```python
from build123d import *

# Parameters (mm, degrees)
F0_W     = 76.2
F0_H     = 76.2
F1_DEPTH = 127
F2_SIZE  = 5.08
F3_R     = 25.4
F4_DEPTH = 25.4
F5_R     = 5.08
F6_DEPTH = 76.2


with BuildPart() as f1:
    # F0 (on Front) → F1 (new body)
    with BuildSketch(Plane.XZ):
        Polygon((12.112662, -9.798872), (-64.087338, -9.798872), (-64.087338, -60.598872), (113.712662, -60.598872), (113.712662, -9.798872), align=None)
        with Locations((-25.987338, 28.301128)):
            Rectangle(F0_W, F0_H)
    extrude(amount=F1_DEPTH)

    # F2
    f2_edges = [f1.edges().sort_by_distance(p)[0] for p in [
        (113.712662, -127, -35.198872),
        (113.712662, 0, -35.198872),
    ]]
    chamfer(f2_edges, length=F2_SIZE)

    # F3 (on face) → F4 (join)
    with BuildSketch(Plane.YZ.offset(12.112662)):
        with Locations((-63.5, 28.301128)):
            Circle(F3_R)
    extrude(amount=F4_DEPTH)

    # F5
    f5_edges = [f1.edges().sort_by_distance(p)[0] for p in [
        (37.512662, -88.9, 28.301128),
    ]]
    fillet(f5_edges, radius=F5_R)

    # F3 (on face) → F6 (join)
    with BuildSketch(Plane.YZ.offset(12.112662)):
        with BuildLine():
            ThreePointArc((-31.75, 85.947037), (-50.392056, 80.668836), (-63.5, 66.401128))
            Line((-63.5, 66.401128), (0, 66.401128))
            ThreePointArc((0, 66.401128), (-13.107944, 80.668836), (-31.75, 85.947037))
        make_face()
        with BuildLine():
            ThreePointArc((-95.25, 85.947037), (-76.607944, 80.668836), (-63.5, 66.401128))
            ThreePointArc((-63.5, 66.401128), (-50.392056, 80.668836), (-31.75, 85.947037))
            ThreePointArc((-31.75, 85.947037), (-63.5, 95.609763), (-95.25, 85.947037))
        make_face()
        with BuildLine():
            Line((-127, 66.401128), (-63.5, 66.401128))
            ThreePointArc((-63.5, 66.401128), (-76.607944, 80.668836), (-95.25, 85.947037))
            ThreePointArc((-95.25, 85.947037), (-113.892056, 80.668836), (-127, 66.401128))
        make_face()
    extrude(amount=-F6_DEPTH)


solid = f1.part
```
Geometry: final body of the model. Coordinates: model frame, mm. Round coordinates to 2 decimals unless told otherwise and drop trailing zeros. Order: outer loops, then holes, each group sorted by start corner. A loop starts at its lowest first (then second) coordinate and runs counter-clockwise, first axis right, second up. Notation, with made-up numbers: (77, 67.25) - (107, 67.25) arc R16 ccw to (107, 82.25) - close; hole circle Ø4 at (1, 33). An arc over 180 degrees is marked (long way). Write item = value, one per line. Start each with the question number.
Q1. Pull-direction query (Z, two-part tool) for faces 1 (the cylindrical face through (-25.45, -113.66, 80.81)), 2 (the cylindrical face through (22.13, -66.807, 53.485)), 3 (the flat face through (37.513, -64, 29)), 4 (the flat face through (24, -63, -60.599)); classes: +Z half, -Z half, draft (parallel to the pull), parting line (faces both ways), or undercut.
Q2. Cut plane A-A on y = -63.5. Return the cut outline in (x, z), and give its area (3 significant figures).
Q3. Cut plane D-D on x = 74. Return the cut outline in (y, z), and give its area (3 significant figures).
Q4. Ray query, line 1 (X direction, y = -73.5, z = -8); line 2 (Z direction, x = 50.5, y = -110); line 3 (X direction, y = -70.5, z = 44). Return the intervals inside material, ascending. Write a range as from..to.
Q5. Pin query (flat end, axial travel): pin 1 (8 mm diameter, centred on y = -92.5, z = -4, fed in from +X); pin 2 (5 mm diameter, centred on x = -10, z = 67.5, fed in from +Y); pin 3 (1 mm diameter, centred on x = -19, y = -76.5, fed in from +Z); pin 4 (4 mm diameter, centred on y = -65, z = 7, fed in from +X). Return the tip coordinate at first contact, or that it passes through.
Q6. Cut plane C-C on y = -100.5. Return the cut outline in (x, z).
Q7. Cut plane B-B on x = -7. Return the cut outline in (y, z).
Outcome:
q1.face_1 = +Z half
q1.face_2 = undercut
q1.face_3 = draft
q1.face_4 = -Z half
q2.outline = (-64.09, -60.6) - (113.71, -60.6) - (113.71, -9.8) - (12.11, -9.8) - (12.11, 2.9) - (32.43, 2.9) arc R5.08 ccw to (37.51, 7.98) - (37.51, 48.62) arc R5.08 ccw to (32.43, 53.7) - (12.11, 53.7) - (12.11, 95.61) - (-64.09, 95.61) - close
q2.area = 18,300 mm^2
q3.outline = (-127, -60.6) - (0, -60.6) - (0, -9.8) - (-127, -9.8) - close
q3.area = 6,450 mm^2
q4.line_1 = -64.09..12.11
q4.line_2 = -60.6..-9.8
q4.line_3 = -64.09..37.51
q5.pin_1 = 12.11
q5.pin_2 = 0
q5.pin_3 = 94.22
q5.pin_4 = 37.51
q6.outline = (-64.09, -60.6) - (113.71, -60.6) - (113.71, -9.8) - (12.11, -9.8) - (12.11, 85.56) - (-64.09, 85.56) - close
q7.outline = (-127, -60.6) - (0, -60.6) - (0, 66.4) arc R35.56 ccw to (-31.75, 85.95) arc R56.99 ccw to (-95.25, 85.95) arc R35.56 ccw to (-127, 66.4) - close
